Autodesk Inventor part; units mm, degrees
ref_plane "YZ Plane" through (0, 0, 0) normal (1, 0, 0) x (0, 1, 0)
ref_plane "XZ Plane" through (0, 0, 0) normal (0, 1, 0) x (-1, 0, 0)
ref_plane "XY Plane" through (0, 0, 0) normal (0, 0, 1) x (1, 0, 0)
sketch "スケッチ1" plane through (0, 0, 0) normal (0, 1, 0) x (-1, 0, 0)
  line L0 (75, 0) -> (105, -51.9615)
  line L1 (-75, 0) -> (-105, -51.9615)
  line L2 (0, -218.2384) -> (0, 36.3731)
  line L3 (147, 0) -> (-147, 0)
  line L4 (105, -51.9615) -> (30, -181.8653)
  line L5 (30, -181.8653) -> (-30, -181.8653)
  line L6 (-30, -181.8653) -> (-105, -51.9615)
  line L7 (75, 0) -> (-75, 0)
  line L8 (34, 0) -> (34, -24.3509)
  line L9 (34, -24.3509) -> (48.7058, -49.822)
  line L10 (48.7058, -49.822) -> (90, -25.9808)
  line L11 (45, 0) -> (45, -18) construction
  line L12 (45, -18) -> (34, -24.3509) construction
  line L13 (84.5, -87.4686) -> (63.4115, -75.2931)
  line L14 (63.4115, -75.2931) -> (48.7058, -49.822)
  line L15 (-34, 0) -> (-34, -24.3509)
  line L16 (-34, -24.3509) -> (-48.7058, -49.822)
  line L17 (-63.4115, -75.2931) -> (-48.7058, -49.822)
  line L18 (-84.5, -87.4686) -> (-63.4115, -75.2931)
  circle A0 centre (30, -32.75) radius 1.6
  circle A1 centre (-30, -32.75) radius 1.6
  line L19 (35.5295, -27) -> (-35.5295, -27)
  point P0 (0, 0)
  point P1 (0, 0)
  point P2 (0, -27)
  dimension "d1" = 150
  dimension "d2" = 60
  dimension "d3" = 60
  dimension "d6" = 60
  dimension "d30" = 60
  dimension "d31" = 18
  dimension "d32" = 30
  dimension "d33" = 41
  dimension "d34" = 3.2
  dimension "d35" = 30
  dimension "d36" = 32.75
  dimension "d37" = 27
extrude "プレート1" add sketch "スケッチ1" along normal blind 1.5 contours L14 L13 L4 L5 L2 L19 L9 | L2 L5 L6 L18 L17 L16 L19
sketch "スケッチ4" plane through (0, 1.5, 0) normal (0, 1, 0) x (1, 0, 0)
  circle A0 centre (30, 67.8013) radius 1.6
  circle A1 centre (45, 67.8013) radius 1.6
  line L0 (0, 218.2384) -> (0, -36.3731)
  circle A2 centre (-30, 67.8013) radius 1.6
  circle A3 centre (-45, 67.8013) radius 1.6
  line L1 (61.6173, 73.1025) -> (25, 73.1025) construction
  line L2 (25, 73.1025) -> (25, 62.5) construction
  line L3 (-61.6173, 73.1025) -> (-25, 73.1025) construction
  line L4 (-25, 73.1025) -> (-25, 62.5) construction
  line L5 (-25, 62.5) -> (25, 62.5)
  line L6 (30, 73.1025) -> (30, 181.8653)
  line L7 (30, 181.8653) -> (-30, 181.8653)
  line L8 (-30, 181.8653) -> (-30, 73.1025)
  line L9 (-25, 62.5) -> (25, 62.5)
  line L10 (25, 62.5) -> (25, 71.0141)
  line L11 (-25, 71.0141) -> (-25, 62.5)
  line L12 (30, 181.8653) -> (84.5, 87.4686)
  line L13 (76.75, 100.892) -> (30, 73.9008)
  line L14 (-30, 73.9008) -> (-76.75, 100.892)
  line L15 (-84.5, 87.4686) -> (-30, 181.8653)
  line L16 (84.5, 87.4686) -> (63.4115, 75.2931)
  line L17 (-63.4115, 75.2931) -> (-84.5, 87.4686)
  line L18 (-35.5295, 27) -> (-63.4115, 75.2931)
  line L19 (62.8673, 70.9375) -> (54.6673, 85.1403)
  arc A4 (54.6673, 85.1403) -> (44.275, 79.1403) centre (49.4712, 82.1403) ccw
  line L20 (44.275, 79.1403) -> (52.475, 64.9375)
  line L21 (52.475, 64.9375) -> (62.8673, 70.9375)
  line L22 (51.2321, 85.1903) -> (52.993, 82.1403)
  line L23 (52.993, 82.1403) -> (51.2321, 79.0903)
  line L24 (51.2321, 79.0903) -> (47.7102, 79.0903)
  line L25 (47.7102, 79.0903) -> (45.9493, 82.1403)
  line L26 (45.9493, 82.1403) -> (47.7102, 85.1903)
  line L27 (47.7102, 85.1903) -> (51.2321, 85.1903)
  line L28 (-30, 73.9008) -> (-25, 71.0141)
  line L29 (30, 73.9008) -> (25, 71.0141)
  point P0 (0, 0)
extrude "切り取り3" cut sketch "スケッチ4" against normal blind 1.5 contours A0 | A1 | L7 L6 L29 L10 L5 L0 | L0 L5 L11 L28 L8 L7 | L12 L13 A4 L6 | L8 L14 L15 | A4 L13 L27 L26 | L26 L27 L13 | A2 | A3
sketch "スケッチ5" plane through (0, 1.5, 0) normal (0, 1, 0) x (1, 0, 0)
  line L0 (-75, 44) -> (75, 44)
  circle A0 centre (-20, 41) radius 3
  circle A1 centre (20, 41) radius 3
  line L1 (-25, 62.5) -> (25, 62.5)
  line L2 (0, 62.5) -> (0, 27)
  line L3 (35.5295, 27) -> (-35.5295, 27)
  circle A2 centre (-20, 41) radius 1.6
  circle A3 centre (20, 41) radius 1.6
  circle A4 centre (0, 37.5) radius 1.6
  point P0 (0, 0)
  dimension "d41" = 6
  dimension "d42" = 6
  dimension "d43" = 40
  dimension "d44" = 3.2
  dimension "d45" = 3.2
  dimension "d46" = 3.2
  dimension "d47" = 3.5
extrude "切り取り4" cut sketch "スケッチ5" against normal blind 1.5 contours A4 L2 | L2 A4 | A2 | A3
sketch "スケッチ6" plane through (0, 1.5, 0) normal (0, 1, 0) x (1, 0, 0)
  ellipse E0 centre (-73.3666, 93.1522) end of major axis (-72.2841, 92.5272) minor radius 1.2133
  circle A0 centre (-48.4391, 79.9279) radius 1.6
  circle A1 centre (-73.3666, 93.1522) radius 1.6
  line L0 (0, 0) -> (0, 20.4537)
  circle A2 centre (48.4391, 79.9279) radius 1.6
  circle A3 centre (73.3666, 93.1522) radius 1.6
  circle A4 centre (-48.4391, 79.9279) radius 1.35
  dimension "d51" = 3.2
  dimension "d52" = 3.2
extrude "切り取り5" cut sketch "スケッチ6" against normal blind 1.5 contours E0 | A0 | A1 | A2 | A3 | A4
fillet "フィレット2" radius 3 12 edges at (-84.5, 0.75, -87.4686) (-76.75, 0.75, -100.892) (-63.4115, 0.75, -75.2931) (-35.5295, 0.75, -27) (35.5295, 0.75, -27) (63.4115, 0.75, -75.2931) (84.5, 0.75, -87.4686) (76.75, 0.75, -100.892) (25, 0.75, -62.5) (-25, 0.75, -62.5) (-25, 0.75, -71.0141) (25, 0.75, -71.0141)
sketch "スケッチ7" plane through (0, 1.5, 0) normal (0, 1, 0) x (1, 0, 0)
  circle A0 centre (-17, 30.5787) radius 1.6
  circle A1 centre (17, 30.5787) radius 1.6
  point P0 (0, 0)
extrude "切り取り6" cut sketch "スケッチ7" against normal blind 1.5
sketch "スケッチ8" plane through (0, 1.5, 0) normal (0, 1, 0) x (1, 0, 0)
  line L0 (37, 32.2376) -> (37, 27.2376) construction
  line L1 (35, 32.2376) -> (37, 32.2376) construction
  line L2 (37, 34.7735) -> (35, 32.2376) construction
  line L3 (38.6077, 34.7735) -> (37, 34.7735) construction
  line L4 (40.6651, 33.5857) -> (38.6077, 34.7735) construction
  line L5 (63.0096, 74.597) -> (36.3955, 28.5)
  line L6 (36.8, 29.2006) -> (36.8, 32.0376)
  line L7 (36.8, 32.0376) -> (34.5875, 32.0376)
  line L8 (34.5875, 32.0376) -> (36.8, 34.8429)
  line L9 (38.8875, 34.8429) -> (39.7651, 34.3362)
  line L10 (36.8, 34.8429) -> (36.903, 34.9735)
  line L11 (36.903, 34.9735) -> (38.6613, 34.9735)
  line L12 (38.6613, 34.9735) -> (38.8876, 34.8428)
  line L13 (39.7651, 34.3362) -> (36.8, 29.2006)
  point P0 (0, 0)
  dimension "d58" = 0.2
  dimension "d59" = 0.2
  dimension "d60" = 0.2
  dimension "d61" = 0.2
  dimension "d62" = 0.2
extrude "押し出し1" cut sketch "スケッチ8" against normal through all
mirror "ミラー1" about plane through (0, 0, 0) normal (1, 0, 0) of "押し出し1"
sketch "スケッチ9" plane through (0, 1.5, 0) normal (0, 1, 0) x (1, 0, 0)
  circle A0 centre (27.3038, 50.6603) radius 1.6
  circle A1 centre (27.3038, 50.6603) radius 5
  point P0 (0, 0)
  dimension "d65" = 10
extrude "切り取り7" cut sketch "スケッチ9" against normal blind 1.5 contours A0 | A1
mirror "ミラー2" about plane through (0, 0, 0) normal (1, 0, 0) of "切り取り7"
equation "\"d3\" = d2"
equation "\"d38\" = Thickness"
equation "\"d41\" = d42"
equation "\"d48\" = Thickness"
equation "\"d53\" = Thickness"
equation "\"d56\" = Thickness"
equation "\"d58\" = d61"
equation "\"d59\" = d61"
equation "\"d60\" = d61"
equation "\"d62\" = d61"
equation "\"d66\" = Thickness"
equation "\"d16\" = Thickness"
properties part number "upper_plate" material "アルミニウム 6061"
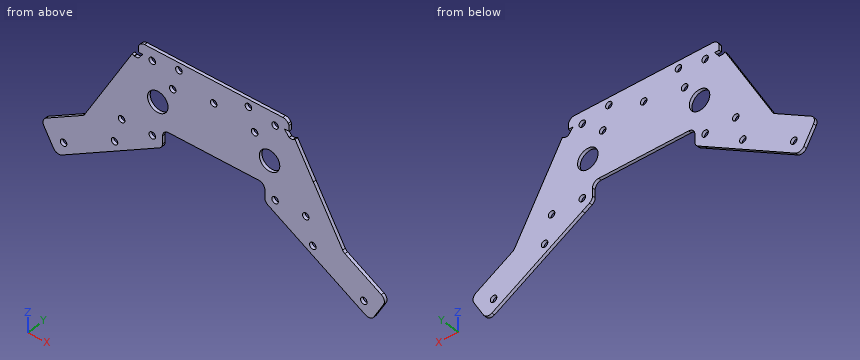
Input: part model. Units: mm. Frame: model coordinates. Give positions to 0.01 mm unless a question says otherwise; leave off trailing zeros. Write each loop counter-clockwise with the first axis right and the second up, starting at its lowest first coordinate (ties: lowest second). Pieces come first, ordered by that corner, then holes. Notation, with made-up numbers: (-4, 68.25) - (18, 68.25) arc R18 cw to (18, 76.25) - close; hole circle Ø4 at (89, 44). An arc over 180 degrees is marked (long way). Write item = value, one per line. Start each with the question number.
1. Ray query, L1, parallel to Z at x = -20, y = 1.1; L2, parallel to X at y = 1.2, z = -31; L3, parallel to Z at x = 0, y = 1.1. Return the intervals inside material, ascending.
2. Section query A-A, the plane z = -37.5. Output: boundary loops of the cut face in (x, y).
3. First-contact query: pin 1 Ø1.9 at (x, z) = (-73.37, -93.15) entering from +Y. Flat tip, straight axial feed; report the tip coordinate or a pass-through.
4. Section query B-B, the plane x = 45. Output: boundary loops of the cut face in (y, z), then the cut area to 3 significant figures.
5. Section query D-D, the plane x = 68. Output: boundary loops of the cut face in (y, z), then the cut area to 3 significant figures.
6. Section query C-C, the plane z = -48. Output: boundary loops of the cut face in (x, y), then the cut area to 3 significant figures.
Check sheet entries:
q1.L1 = -62.5 to -42.6, -39.4 to -27
q1.L2 = -36.8 to -18.54, -15.46 to 15.46, 18.54 to 36.8
q1.L3 = -62.5 to -39.1, -35.9 to -27
q2.outline = (-41.59, 0) - (-1.6, 0) - (-1.6, 1.5) - (-41.59, 1.5) - close; (1.6, 0) - (41.59, 0) - (41.59, 1.5) - (1.6, 1.5) - close
q3.pin_1 = through
q4.outline = (0, -82.56) - (1.5, -82.56) - (1.5, -69.4) - (0, -69.4) - close; (0, -66.2) - (1.5, -66.2) - (1.5, -43.4) - (0, -43.4) - close
q4.area = 53.9 mm2
q5.outline = (0, -95.84) - (1.5, -95.84) - (1.5, -77.94) - (0, -77.94) - close
q5.area = 26.8 mm2
q6.outline = (-47.65, 0) - (-31.54, 0) - (-31.54, 1.5) - (-47.65, 1.5) - close; (-23.07, 0) - (23.07, 0) - (23.07, 1.5) - (-23.07, 1.5) - close; (31.54, 0) - (47.65, 0) - (47.65, 1.5) - (31.54, 1.5) - close
q6.area = 118 mm2
